```python
from build123d import *

# Parameters (mm, degrees)
F0_W     = 3.175
F0_H     = 76.2
F1_DEPTH = 1.190625
F2_DEPTH = 16.51
F3_START = -12.7
F3_DEPTH = 3.81


# Not quite as in the source:
# - a length typed as a fraction of an inch, garbled in the dataset ("3 / 203.2 mm" for 3/8 in), is restored


with BuildPart() as f1:
    # F0 (on Top) → F1 (new body)
    with BuildSketch(Plane.XY):
        with Locations((-34.925, 0)):
            Rectangle(F0_W, F0_H)
        with BuildLine():
            Line((-30.1625, 38.1), (-30.1625, -38.1))
            Line((-30.1625, -38.1), (0, -38.1))
            Line((0, -38.1), (0, -31.8450108171))
            Line((0, -31.8450108171), (-2.553815411, -31.8450108171))
            ThreePointArc((-2.553815411, -31.8450108171), (-7.0439434716, -29.9851388776), (-8.903815411, -25.4950108171))
            Line((-8.903815411, -25.4950108171), (-8.903815411, 25.3049891829))
            ThreePointArc((-8.903815411, 25.3049891829), (-7.0439434716, 29.7951172435), (-2.553815411, 31.6549891829))
            Line((-2.553815411, 31.6549891829), (0, 31.6549891829))
            Line((0, 31.6549891829), (0, 38.1))
            Line((0, 38.1), (-30.1625, 38.1))
        make_face()
        with Locations((-31.75, 0)):
            Rectangle(F0_W, F0_H)
    extrude(amount=F1_DEPTH)

    # F0 (on Top) → F2 (join)
    with BuildSketch(Plane.XY):
        with Locations((-34.925, 0)):
            Rectangle(F0_W, F0_H)
    extrude(amount=-F2_DEPTH)

    # F0 (on Top) → F3 (join)
    with BuildSketch(Plane.XY.offset(F3_START)):
        with Locations((-34.925, 0)):
            Rectangle(F0_W, F0_H)
        with Locations((-31.75, 0)):
            Rectangle(F0_W, F0_H)
    extrude(amount=-F3_DEPTH)


solid = f1.part
```
CAD build for the part. Positions are in the model's coordinates, mm. A direction names the side the tool comes from. Round coordinates to 2 decimals unless told otherwise and drop trailing zeros. Order: outer loops, then holes, each group sorted by start corner. A loop starts at its lowest first (then second) coordinate and runs counter-clockwise, first axis right, second up.
Q1. Slice it at D-D (z = -8). Write the cut outline in (x, y).
Q2. Two-plate mould, pull along Y, no slides. Class faces 4 (the flat face through (-33.338, -1, -6)), 5 (the flat face through (-27.8, 38.1, 0.2)), 6 (the cylindrical face through (-7.09, 29.75, 0.59)): pulls with the +Y half, pulls with the -Y half, needs draft (parallel to the pull), parting line crosses it, or undercut.
Q3. Wall check: L1, parallel to Z at x = -32, y = -18.5; L2, parallel to Z at x = -16, y = -9; L3, parallel to X at y = 0, z = -9.5. Give the ranges that are in metal, low to high.
Q4. Slice it at C-C (x = -11). Write the cut outline in (y, z), and give its area (3 significant figures).
Q5. Slice it at B-B (y = 8). Write the cut outline in (x, z).
Q6. Which spindle directions (+Z, -Z, +X, -X, +Y, -Y) get a long thin tool onto all of the face, cutting with end or side? Do faces 1 (the cylindrical face through (-6.994, -30.034, 0.587)), 2 (the flat face through (-21, 1, 0)), 3 (the flat face through (-30.162, -1, -15)). Say none if no direction does.
Q7. Drop flat-ended pins along their axis: pin 1 (1 mm diameter, centred on x = -4.5, y = 30, fed in from -Z); pin 2 (5 mm diameter, centred on x = -14, y = 8.5, fed in from -Z); pin 3 (3 mm diameter, centred on y = 2, z = -15, fed in from +X); pin 4 (0.6 mm diameter, centred on y = -12.5, z = 1, fed in from +X). Give the stop position or say it passes through.
Q8. Slice it at A-A (x = -7). Write the cut outline in (y, z), and give its area (3 significant figures).
Results below:
1. outline: (-36.51, -38.1) - (-33.34, -38.1) - (-33.34, 38.1) - (-36.51, 38.1) - close
2. face 4: needs draft
2. face 5: pulls with the +Y half
2. face 6: undercut
3. L1: z = -16.51 to -12.7, 0 to 1.19
3. L2: z = 0 to 1.19
3. L3: x = -36.51 to -33.34
4. outline: (-38.1, 0) - (38.1, 0) - (38.1, 1.19) - (-38.1, 1.19) - close
4. area: 90.7 mm2
5. outline: (-36.51, -16.51) - (-30.16, -16.51) - (-30.16, -12.7) - (-33.34, -12.7) - (-33.34, 0) - (-8.9, 0) - (-8.9, 1.19) - (-36.51, 1.19) - close
6. face 1: +Z, -Z, +X
6. face 2: +X, +Y, -Y
6. face 3: -Z, +X, +Y, -Y
7. pin 1: passes through
7. pin 2: stops at z = 0
7. pin 3: stops at x = -30.16
7. pin 4: stops at x = -8.9
8. outline: (-38.1, 0) - (-30.03, 0) - (-30.03, 1.19) - (-38.1, 1.19) - close; (29.84, 0) - (38.1, 0) - (38.1, 1.19) - (29.84, 1.19) - close
8. area: 19.4 mm2
